Autodesk Inventor part; units mm, degrees
ref_plane "YZ Plane" through (0, 0, 0) normal (1, 0, 0) x (0, 1, 0)
ref_plane "XZ Plane" through (0, 0, 0) normal (0, 1, 0) x (-1, 0, 0)
ref_plane "XY Plane" through (0, 0, 0) normal (0, 0, 1) x (1, 0, 0)
sketch "Эскиз1" plane through (0, 0, 0) normal (0, 0, 1) x (1, 0, 0)
  circle A0 centre (0, 0) radius 10.025
  dimension "d0" = 20.05
extrude "Выдавливание1" add sketch "Эскиз1" along normal blind 21.5
sketch "Эскиз2" plane through (0, 0, 21.5) normal (0, 0, 1) x (1, 0, 0)
  circle A0 centre (0, 0) radius 5
  dimension "d3" = 10
extrude "Выдавливание2" add sketch "Эскиз2" along normal blind 2
sketch "Эскиз3" plane through (0, 0, 0) normal (0, 0, -1) x (-1, 0, 0)
  circle A0 centre (0, 0) radius 10
  line L0 (6.3804, -7.7) -> (-6.4196, -7.7)
  circle A1 centre (0, 0) radius 10.025 construction
  line L1 (-10.025, 0) -> (10.025, 0) construction
  circle A2 centre (0, 0) radius 10.025 construction
  line L2 (6.3804, 7.7) -> (-6.4196, 7.7)
  point P0 (-6.3804, 7.7)
  point P1 (-6.3804, -7.7)
  dimension "d6" = 20
  dimension "d10" = 15.4
extrude "Выдавливание3" add sketch "Эскиз3" along normal blind 32 contours A0 L0 L2
sketch "Эскиз4" plane through (0, 0, 21.5) normal (0, 0, 1) x (1, 0, 0)
  circle A0 centre (0, 0) radius 7.5 construction
  circle A1 centre (1.9411, 7.2444) radius 1.25
  circle A2 centre (0, 0) radius 10.025 construction
  line L0 (0, 10.025) -> (0, -10.025) construction
  line L1 (1.9411, 7.2444) -> (0, 0) construction
  circle A3 centre (-7.2444, -1.9411) radius 1.25
  circle A4 centre (5.3033, -5.3033) radius 1.25
  dimension "d11" = 15
  dimension "d12" = 2.5
  dimension "d13" = 15
  dimension "d16" = 360
extrude "Выдавливание4" cut sketch "Эскиз4" against normal blind 5
sketch "Эскиз5" plane through (0, 0, -32) normal (0, 0, -1) x (-1, 0, 0)
  circle A0 centre (0, 0) radius 3.1
  dimension "d20" = 6.2
extrude "Выдавливание5" add sketch "Эскиз5" along normal blind 2.1
fillet "Сопряжение1" radius 0.5 1 edges at (3.1, 0, -34.1)
sketch "Эскиз6" plane through (0, 0, -34.1) normal (0, 0, -1) x (-1, 0, 0)
  circle A0 centre (0, 0) radius 1
  dimension "d24" = 2
extrude "Выдавливание6" add sketch "Эскиз6" along normal blind 4.1
sketch "Эскиз7" plane through (0, 0, 23.5) normal (0, 0, 1) x (1, 0, 0)
  circle A0 centre (0, 0) radius 2
  dimension "d27" = 4
extrude "Выдавливание7" cut sketch "Эскиз7" against normal blind 10
properties part number "motor_body"
For this review, take the finished solid that the model builds, in its own axes (mm). A direction names the side the tool comes from. Round coordinates to 2 decimals unless told otherwise and drop trailing zeros. Loops run counter-clockwise (first coordinate to the right, second up) from the corner with the lowest first, then second, coordinate; pieces in that order, holes last. Notation, with made-up numbers: (61, -11) - (100, -11) arc R29 ccw to (100, 16) - close; hole circle Ø4 at (52, 68.25). An arc over 180 degrees is marked (long way). Use one line per item in the form item = value.
Item 1: Mouldability with a two-part tool opening along X and no side actions: class faces 1 (the flat face through (-5, -2, 21.5)), 2 (the cylindrical face through (-8.493, -1.886, 19.035)), 3 (the cylindrical face through (-10, 0, -16)) as +X half, -X half, draft (parallel to the pull), parting line (faces both ways), or undercut.
Answers:
face_1 = draft
face_2 = undercut
face_3 = -X half
Item 2: Consider section D-D on z = 3. Write out the cut boundary in (x, y) (3 decimals), then the cut area to 3 significant figures.
Answers:
outline = circle Ø20.05 at (0, 0)
area = 316 mm^2
Item 3: Consider section B-B on z = 15. Write out the cut boundary in (x, y) (3 decimals), then the cut area to 3 significant figures.
Answers:
outline = circle Ø20.05 at (0, 0); hole circle Ø4 at (0, 0)
area = 303 mm^2
Item 4: For line 1 (Y direction, x = 0, z = 19.5) (3 decimals); line 2 (Y direction, x = 1.5, z = -2.5); line 3 (Z direction, x = -7.25, y = 0.75), list the stretches that pass through material, from the lowest coordinate up.
Answers:
line_1 = -10.025 to -2, 2 to 10.025
line_2 = -7.7 to 7.7
line_3 = -32 to 21.5
Item 5: Consider section A-A on y = 0. Write out the cut boundary in (x, z) (3 decimals), then the cut area to 3 significant figures.
Answers:
outline = (-10.025, 0) - (-10, 0) - (-10, -32) - (-3.1, -32) - (-3.1, -33.6) arc R0.5 ccw to (-2.6, -34.1) - (-1, -34.1) - (-1, -38.2) - (1, -38.2) - (1, -34.1) - (2.6, -34.1) arc R0.5 ccw to (3.1, -33.6) - (3.1, -32) - (10, -32) - (10, 0) - (10.025, 0) - (10.025, 21.5) - (5, 21.5) - (5, 23.5) - (2, 23.5) - (2, 13.5) - (-2, 13.5) - (-2, 23.5) - (-5, 23.5) - (-5, 21.5) - (-10.025, 21.5) - close
area = 1,070 mm^2
Item 6: Consider section C-C on x = 0. Write out the cut boundary in (y, z) (3 decimals).
Answers:
outline = (-10.025, 0) - (-7.7, 0) - (-7.7, -32) - (-3.1, -32) - (-3.1, -33.6) arc R0.5 ccw to (-2.6, -34.1) - (-1, -34.1) - (-1, -38.2) - (1, -38.2) - (1, -34.1) - (2.6, -34.1) arc R0.5 ccw to (3.1, -33.6) - (3.1, -32) - (7.7, -32) - (7.7, 0) - (10.025, 0) - (10.025, 21.5) - (5, 21.5) - (5, 23.5) - (2, 23.5) - (2, 13.5) - (-2, 13.5) - (-2, 23.5) - (-5, 23.5) - (-5, 21.5) - (-10.025, 21.5) - close
Item 7: Clearance check with flat-ended pins moving along their axes: P1, Ø4, axis at y = 7.5, z = -14, coming from the +X side; P2, Ø5, axis at x = 6, z = 5.5, coming from the +Y side; P3, Ø2, axis at x = 5.3, y = -5.3, coming from the -Z side. State where each tip first meets the part, or that it passes through.
Answers:
P1 = 8.35
P2 = 9.39
P3 = -32
Item 8: Tool access review of faces 4 (the flat face through (0, -7.7, -16)), 5 (the flat face through (0, 4, -32)), 6 (the flat face through (0, 0, -38.2)), 7 (the cylindrical face through (-1.08, 4.88, 22.49)): name each direction out of +Z, -Z, +X, -X, +Y, -Y from which nothing blocks a thin tool from reaching the whole face with its end or side.
Answers:
face_4 = -Z, +X, -X, -Y
face_5 = -Z
face_6 = -Z, +X, -X, +Y, -Y
face_7 = +Z
